The model under review builds one solid part; all positions refer to its coordinate system, in mm. A direction names the side the tool comes from. Give positions to 0.01 mm unless a question says otherwise; leave off trailing zeros. Order: outer loops, then holes, each group sorted by start corner. A loop starts at its lowest first (then second) coordinate and runs counter-clockwise, first axis right, second up.
```python
from build123d import *

# Parameters (mm, degrees)
SKETCH1_W           = 180
SKETCH1_H           = 240
BOSS_EXTRUDE1_DEPTH = 5
SKETCH2_R           = 3.6
SKETCH2_W           = 40.55
SKETCH2_H           = 34.5
CUT_EXTRUDE1_DEPTH  = 6
SKETCH3_W           = 12.5
SKETCH3_H           = 12.5
CUT_EXTRUDE2_DEPTH  = 2.5
SKETCH4_W           = 35.55
SKETCH4_H           = 8
CUT_EXTRUDE3_DEPTH  = 2.5
FILLET1_R           = 10
BOSS_EXTRUDE2_DEPTH = 9.5
FILLET2_R           = 2


with BuildPart() as part:
    # Sketch1 → Boss-Extrude1 (new body)
    with BuildSketch(Plane(origin=(0, 0, 0), x_dir=(1, 0, 0), z_dir=(0, 1, 0))):
        with Locations((90, 120)):
            Rectangle(SKETCH1_W, SKETCH1_H)
    extrude(amount=BOSS_EXTRUDE1_DEPTH)

    # Sketch2 → Cut-Extrude1 (cut, through all)
    with BuildSketch(Plane.XZ):
        with Locations((105.55, -215)):
            Circle(SKETCH2_R)
        with Locations((60.275, -207.75)):
            Rectangle(SKETCH2_W, SKETCH2_H)
    extrude(amount=-CUT_EXTRUDE1_DEPTH, mode=Mode.SUBTRACT)

    # Sketch3 → Cut-Extrude2 (cut)
    with BuildSketch(Plane(origin=(0, 5, 0), x_dir=(1, 0, 0), z_dir=(0, 1, 0))):
        with Locations((105.55, 215)):
            Rectangle(SKETCH3_W, SKETCH3_H)
    extrude(amount=-CUT_EXTRUDE2_DEPTH, mode=Mode.SUBTRACT)

    # Sketch4 → Cut-Extrude3 (cut)
    with BuildSketch(Plane(origin=(0, 5, 0), x_dir=(1, 0, 0), z_dir=(0, 1, 0))):
        with Locations((60.275, 186.5)):
            Rectangle(SKETCH4_W, SKETCH4_H)
    extrude(amount=-CUT_EXTRUDE3_DEPTH, mode=Mode.SUBTRACT)

    # Fillet1
    fillet1_edges = [part.edges().sort_by_distance(p)[0] for p in [
        (0, 2.5, -240),
        (180, 2.5, -240),
        (180, 2.5, 0),
        (0, 2.5, 0),
    ]]
    fillet(fillet1_edges, radius=FILLET1_R)

    # Sketch6 → Boss-Extrude2 (add)
    with BuildSketch(Plane(origin=(0, 5, 0), x_dir=(1, 0, 0), z_dir=(0, 1, 0))):
        with BuildLine():
            Line((175.7, 10), (175.7, 230))
            ThreePointArc((175.7, 230), (174.030508653, 234.030508653), (170, 235.7))
            Line((170, 235.7), (10, 235.7))
            ThreePointArc((10, 235.7), (5.969491347, 234.030508653), (4.3, 230))
            Line((4.3, 230), (4.3, 10))
            ThreePointArc((4.3, 10), (5.969491347, 5.969491347), (10, 4.3))
            Line((10, 4.3), (170, 4.3))
            ThreePointArc((170, 4.3), (174.030508653, 5.969491347), (175.7, 10))
        make_face()
        with BuildLine():
            Line((170.7, 10), (170.7, 230))
            ThreePointArc((170.7, 230), (170.494974747, 230.494974747), (170, 230.7))
            Line((170, 230.7), (10, 230.7))
            ThreePointArc((10, 230.7), (9.505025253, 230.494974747), (9.3, 230))
            Line((9.3, 230), (9.3, 10))
            ThreePointArc((9.3, 10), (9.505025253, 9.505025253), (10, 9.3))
            Line((10, 9.3), (170, 9.3))
            ThreePointArc((170, 9.3), (170.494974747, 9.505025253), (170.7, 10))
        make_face(mode=Mode.SUBTRACT)
    extrude(amount=BOSS_EXTRUDE2_DEPTH)

    # Fillet2
    fillet2_edges = [part.edges().sort_by_distance(p)[0] for p in [
        (174.030508653, 14.5, -5.969491347),
        (175.7, 14.5, -120),
        (174.030508653, 14.5, -234.030508653),
        (90, 14.5, -235.7),
        (5.969491347, 14.5, -234.030508653),
        (4.3, 14.5, -120),
        (5.969491347, 14.5, -5.969491347),
        (90, 14.5, -4.3),
    ]]
    fillet(fillet2_edges, radius=FILLET2_R)


solid = part.part
```
Item 1: For line 1 (X direction, y = 0.6, z = -215); line 2 (Z direction, x = 105.55, y = 0.8); line 3 (X direction, y = 10, z = -188), list the stretches that pass through material, from the lowest coordinate up.
Values found:
line 1: x = 0 to 40, 80.55 to 101.95, 109.15 to 180
line 2: z = -240 to -218.6, -211.4 to 0
line 3: x = 4.3 to 9.3, 170.7 to 175.7
Item 2: Take a section at D-D (z = -82.5). Give the boundary of the cut face in (x, y).
Values found:
outline: (0, 0) - (180, 0) - (180, 5) - (175.7, 5) - (175.7, 12.5) arc R2 ccw to (173.7, 14.5) - (170.7, 14.5) - (170.7, 5) - (9.3, 5) - (9.3, 14.5) - (6.3, 14.5) arc R2 ccw to (4.3, 12.5) - (4.3, 5) - (0, 5) - close
Item 3: For faces 3 (the flat face through (60, 2.5, -187)), 4 (the cylindrical face through (173.99, 8.7, -5.93)), 5 (the flat face through (91, 9, -235.7)), 6 (the flat face through (89, 9, -4.3)), 7 (the flat face through (4.3, 9, -122)), list the 3-axis set-ups (+Z, -Z, +X, -X, +Y, -Y) from which the entire face can be reached by the end or side of a thin tool; tool diameter is ignored.
Values found:
face 3: +Y
face 4: +Z, +X, +Y
face 5: -Z, +X, -X, +Y
face 6: +Z, +X, -X, +Y
face 7: +Z, -Z, -X, +Y
Item 4: Take a section at B-B (z = -215). Give the boundary of the cut face in (x, y), and give its area (3 significant figures).
Values found:
outline: (0, 0) - (40, 0) - (40, 5) - (9.3, 5) - (9.3, 14.5) - (6.3, 14.5) arc R2 ccw to (4.3, 12.5) - (4.3, 5) - (0, 5) - close; (80.55, 0) - (101.95, 0) - (101.95, 2.5) - (99.3, 2.5) - (99.3, 5) - (80.55, 5) - close; (109.15, 0) - (180, 0) - (180, 5) - (175.7, 5) - (175.7, 12.5) arc R2 ccw to (173.7, 14.5) - (170.7, 14.5) - (170.7, 5) - (111.8, 5) - (111.8, 2.5) - (109.15, 2.5) - close
area: 741 mm2
Item 5: Clearance check with flat-ended pins moving along their axes: pin 1 Ø6 at (x, z) = (106.5, -135) entering from +Y; pin 2 Ø5 at (y, z) = (9, -179.5) entering from -X; pin 3 Ø4 at (y, z) = (8, -169.5) entering from +X. State where each tip first meets the part, or that it passes through.
Values found:
pin 1: stops at y = 5
pin 2: stops at x = 4.3
pin 3: stops at x = 175.7
Item 6: Take a section at A-A (x = 105.55). Give the boundary of the cut face in (y, z).
Values found:
outline: (0, -240) - (5, -240) - (5, -235.7) - (12.5, -235.7) arc R2 ccw to (14.5, -233.7) - (14.5, -230.7) - (5, -230.7) - (5, -221.25) - (2.5, -221.25) - (2.5, -218.6) - (0, -218.6) - close; (0, -211.4) - (2.5, -211.4) - (2.5, -208.75) - (5, -208.75) - (5, -9.3) - (14.5, -9.3) - (14.5, -6.3) arc R2 ccw to (12.5, -4.3) - (5, -4.3) - (5, 0) - (0, 0) - close
Item 7: Take a section at C-C (x = 34.5). Give the boundary of the cut face in (y, z), and give its area (3 significant figures).
Values found:
outline: (0, -240) - (5, -240) - (5, -235.7) - (12.5, -235.7) arc R2 ccw to (14.5, -233.7) - (14.5, -230.7) - (5, -230.7) - (5, -9.3) - (14.5, -9.3) - (14.5, -6.3) arc R2 ccw to (12.5, -4.3) - (5, -4.3) - (5, 0) - (0, 0) - close
area: 1,290 mm2
Item 8: Draft analysis for pull direction Y (two halves, no side actions). For faces 1 (the flat face through (80.55, 2, -208)), 2 (the flat face through (9, 14.5, -121)), state which applies: released by +Y, released by -Y, zero draft, split by the parting line, or undercut.
Values found:
face 1: zero draft
face 2: released by +Y
